Source: CAD feature listing. Evaluate the final solid. Frame: model axes, mm. Give positions to 0.01 mm unless a question says otherwise; leave off trailing zeros. Order: outer loops, then holes, each group sorted by start corner. A loop starts at its lowest first (then second) coordinate and runs counter-clockwise, first axis right, second up. Notation, with made-up numbers: M 5,37.5 L 13,37.5 A32 cw 13,64.5 Z; hole C 72,54 d9. An arc over 180 degrees is marked long. Answer as a JSON object with one key per item and string values. Group by question number.
1. Section query A-A (x = -42). Output: boundary loops of the cut face in (y, z), plus the area to 3 significant figures.
2. Material intervals for L1, parallel to X at y = -190, z = 0.85; L2, parallel to Y at x = 6, z = 2.4, sorted ascending. Write a range as [from, to].
3. Pull-direction query (Z, two-part tool) for faces 1 (the flat face through (-181, 3, 3)), 2 (the flat face through (-181, 3, 0)); classes: +Z half, -Z half, draft (parallel to the pull), parting line (faces both ways), or undercut.
4. Section query C-C (z = 0.85). Output: boundary loops of the cut face in (x, y), plus the area to 3 significant figures.
from build123d import *

# Parameters (mm, degrees)
ESQUISSE1_W        = 400
ESQUISSE1_H        = 400
ESQUISSE1_W_2      = 340
ESQUISSE1_H_2      = 340
BOSS_EXTRU_1_DEPTH = 3
D_GAGEMENT_M51_D   = 5.5


with BuildPart() as part:
    # Esquisse1 → Boss.-Extru.1 (new body)
    with BuildSketch(Plane.XY):
        Rectangle(ESQUISSE1_W, ESQUISSE1_H)
        Rectangle(ESQUISSE1_W_2, ESQUISSE1_H_2, mode=Mode.SUBTRACT)
    extrude(amount=BOSS_EXTRU_1_DEPTH)

    # Dégagement M51 (through all)
    with Locations(Plane.XY.offset(3)):
        with Locations((-190, -190), (-190, 190), (190, 190), (190, -190)):
            Hole(D_GAGEMENT_M51_D / 2)


solid = part.part
Answer sheet:
{
 "1": {"outline": "M -200,0 L -170,0 L -170,3 L -200,3 Z; M 170,0 L 200,0 L 200,3 L 170,3 Z", "area": "180 mm^2"},
 "2": {"L1": "[-200, -192.75], [-187.25, 187.25], [192.75, 200]", "L2": "[-200, -170], [170, 200]"},
 "3": {"face 1": "+Z half", "face 2": "-Z half"},
 "4": {"outline": "M -200,-200 L 200,-200 L 200,200 L -200,200 Z; hole C -190,-190 d5.5; hole C -190,190 d5.5; hole M -170,-170 L 170,-170 L 170,170 L -170,170 Z; hole C 190,-190 d5.5; hole C 190,190 d5.5", "area": "44,300 mm^2"}
}
